Check sheet for the modelled part. Datum: model origin and axes. Units: mm. Face numbers are marked on the shaded views. Round coordinates to 2 decimals unless told otherwise and drop trailing zeros. Write each loop counter-clockwise with the first axis right and the second up, starting at its lowest first coordinate (ties: lowest second). Pieces come first, ordered by that corner, then holes. Notation, with made-up numbers: (-29.5, 81) -> (-9.5, 81) arc R27 ccw to (-9.5, 112) -> close; hole circle Ø11 at (77, -39). An arc over 180 degrees is marked (long way). Put each result on its own line as item: value. Start each with the question number.
from build123d import *

# Parameters (mm, degrees)
SKETCH1_R           = 30
BOSS_EXTRUDE1_DEPTH = 3.54
BOSS_EXTRUDE4_START = -3
BOSS_EXTRUDE4_DEPTH = 3
CUT_EXTRUDE3_DEPTH  = 6
BOSS_EXTRUDE5_DEPTH = 6
BOSS_EXTRUDE6_DEPTH = 0.4
CUT_EXTRUDE4_REACH  = 71.98
SKETCH12_R          = 2


with BuildPart() as part:
    # Sketch1 → Boss-Extrude1 (new body)
    with BuildSketch(Plane.XY):
        Circle(SKETCH1_R)
    extrude(amount=BOSS_EXTRUDE1_DEPTH)

    # Sketch4 → Boss-Extrude4 (add)
    with BuildSketch(Plane.XY.offset(3.54).offset(BOSS_EXTRUDE4_START)):
        with BuildLine():
            Line((25.054939633, 16.5), (70, 16.5))
            Line((70, 16.5), (70, -16.5))
            Line((70, -16.5), (25.054939633, -16.5))
            ThreePointArc((25.054939633, -16.5), (30, 0), (25.054939633, 16.5))
        make_face()
    extrude(amount=BOSS_EXTRUDE4_DEPTH)

    # Sketch9 → Cut-Extrude3 (cut)
    with BuildSketch(Plane(origin=(0, 0, 0), x_dir=(-1, 0, 0), z_dir=(0, 0, -1))):
        Polygon((0, 5.773502692), (-5, 2.886751346), (-5, -2.886751346), (0, -5.773502692), (5, -2.886751346), (5, 2.886751346), align=None)
    extrude(amount=-CUT_EXTRUDE3_DEPTH, mode=Mode.SUBTRACT)

    # Sketch10 → Boss-Extrude5 (add)
    with BuildSketch(Plane.XY.offset(3.54)):
        Polygon((0, 8.660254038), (-7.5, 4.330127019), (-7.5, -4.330127019), (0, -8.660254038), (7.5, -4.330127019), (7.5, 4.330127019), align=None)
        Polygon((0, 5.773502692), (-5, 2.886751346), (-5, -2.886751346), (0, -5.773502692), (5, -2.886751346), (5, 2.886751346), align=None, mode=Mode.SUBTRACT)
    extrude(amount=BOSS_EXTRUDE5_DEPTH)

    # Sketch11 → Boss-Extrude6 (add)
    with BuildSketch(Plane.XY.offset(9.54)):
        Polygon((0, 5.773502692), (-5, 2.886751346), (-5, -2.886751346), (0, -5.773502692), (5, -2.886751346), (5, 2.886751346), align=None)
    extrude(amount=-BOSS_EXTRUDE6_DEPTH)

    # Sketch12 → Cut-Extrude4 (cut, up to next)
    with BuildSketch(Plane(origin=(7.5, 0, 0), x_dir=(0, 0, -1), z_dir=(1, 0, 0)), mode=Mode.PRIVATE) as cut_extrude4_sk1:
        with Locations((-6, 0)):
            Circle(SKETCH12_R)
    cut_extrude4_tool1 = extrude(cut_extrude4_sk1.sketch, amount=-CUT_EXTRUDE4_REACH, mode=Mode.PRIVATE) & part.part
    add(cut_extrude4_tool1.solids().sort_by_distance((7.5, 0, 6))[0], mode=Mode.SUBTRACT)


solid = part.part
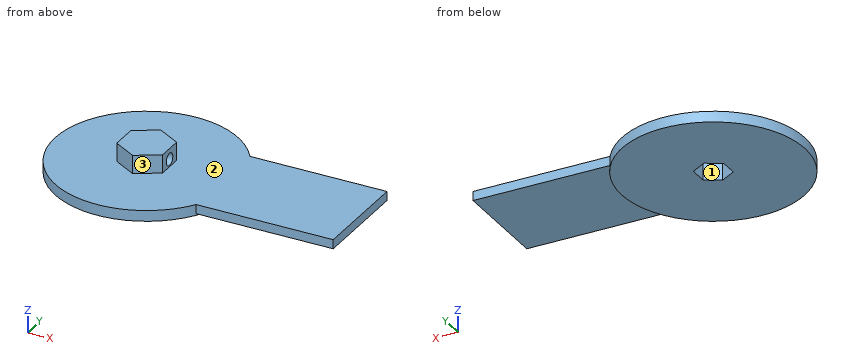
1. Section check B-B, the plane y = 0. Enter the section's corners in (x, z).
2. Gauge pin test, flat ends, axial feed: P1, Ø1.8, axis at y = 2, z = 5.5, coming from the +X side; P2, Ø3, axis at y = 18.5, z = 2.5, coming from the -X side; P3, Ø2.5, axis at x = 51.5, z = 1.5, coming from the -Y side; P4, Ø1, axis at x = 17.5, z = 5.5, coming from the -Y side. Record the tip position at first contact, or that the pin passes through.
3. Material ranges on L1, parallel to X at y = -0.5, z = 3; L2, parallel to X at y = 0.5, z = 5.75; L3, parallel to X at y = -3.5, z = 2, recorded low to high. Write a range as [from, to].
4. Section check C-C, the plane x = 28.5. Enter the section's corners in (y, z).
5. Section check A-A, the plane z = 6. Enter the section's corners in (x, y).
6. Section check D-D, the plane y = -24. Enter the section's corners in (x, z).
7. Draft check along X on the marked faces 1, 2 and 3. Enter one of: released by +X, released by -X, zero draft, split by the parting line, or undercut.
Reply:
1. outline: (-30, 0) -> (-5, 0) -> (-5, 9.14) -> (5, 9.14) -> (5, 8) -> (7.5, 8) -> (7.5, 9.54) -> (-7.5, 9.54) -> (-7.5, 3.54) -> (-30, 3.54) -> close; (5, 0) -> (30, 0) -> (30, 0.54) -> (70, 0.54) -> (70, 3.54) -> (7.5, 3.54) -> (7.5, 4) -> (5, 4) -> close
2. P1: stops at x = 7.5
2. P2: stops at x = -24.72
2. P3: stops at y = -16.5
2. P4: passes through
3. L1: x = [-30, -5], [5, 70]
3. L2: x = [-7.5, -5]
3. L3: x = [-29.8, -3.94], [3.94, 70]
4. outline: (-16.5, 0.54) -> (-9.37, 0.54) -> (-9.37, 0) -> (9.37, 0) -> (9.37, 0.54) -> (16.5, 0.54) -> (16.5, 3.54) -> (-16.5, 3.54) -> close
5. outline: (-7.5, -4.33) -> (0, -8.66) -> (7.5, -4.33) -> (7.5, -2) -> (5, -2) -> (5, -2.89) -> (0, -5.77) -> (-5, -2.89) -> (-5, 2.89) -> (0, 5.77) -> (5, 2.89) -> (5, 2) -> (7.5, 2) -> (7.5, 4.33) -> (0, 8.66) -> (-7.5, 4.33) -> close
6. outline: (-18, 0) -> (18, 0) -> (18, 3.54) -> (-18, 3.54) -> close
7. face 1: undercut
7. face 2: zero draft
7. face 3: released by +X
